```python
from build123d import *

# Parameters (mm, degrees)
SKETCH1_W                                            = 45
SKETCH1_H                                            = 50
SKETCH1_R                                            = 1.5
SKETCH1_R_2                                          = 2.5
BOSS_EXTRUDE1_DEPTH                                  = 20
SKETCH3_W                                            = 26
SKETCH3_H                                            = 28
CUT_EXTRUDE1_DEPTH                                   = 10
REFRENTADO_PARA_TORNILLO_CON_CABEZA_PLAN_D           = 3.2
REFRENTADO_PARA_TORNILLO_CON_CABEZA_PLAN_CBORE_D     = 6.5
REFRENTADO_PARA_TORNILLO_CON_CABEZA_PLAN_CBORE_DEPTH = 2
FILLET4_R                                            = 5
BOSS_EXTRUDE4_DEPTH                                  = 50
FILLET5_R                                            = 4.5
FILLET6_R                                            = 2.5


with BuildPart() as part:
    # Sketch1 → Boss-Extrude1 (new body)
    with BuildSketch(Plane(origin=(0, 0, 0), x_dir=(1, 0, 0), z_dir=(0, 1, 0))):
        Rectangle(SKETCH1_W, SKETCH1_H)
        with Locations(Location((-7.5, 8, 0), (0, 0, 270))):
            Circle(SKETCH1_R, mode=Mode.SUBTRACT)
        with Locations(Location((7.5, 8, 0), (0, 0, 270))):
            Circle(SKETCH1_R, mode=Mode.SUBTRACT)
        with Locations(Location((7.5, -8, 0), (0, 0, 270))):
            Circle(SKETCH1_R, mode=Mode.SUBTRACT)
        with Locations(Location((-7.5, -8, 0), (0, 0, 270))):
            Circle(SKETCH1_R, mode=Mode.SUBTRACT)
        with Locations(Location((15.3, 17, 0), (0, 0, 270))):
            Circle(SKETCH1_R_2, mode=Mode.SUBTRACT)
        with Locations(Location((-15.3, 17, 0), (0, 0, 270))):
            Circle(SKETCH1_R_2, mode=Mode.SUBTRACT)
        with Locations(Location((-15.3, -17, 0), (0, 0, 270))):
            Circle(SKETCH1_R_2, mode=Mode.SUBTRACT)
        with Locations(Location((15.3, -17, 0), (0, 0, 270))):
            Circle(SKETCH1_R_2, mode=Mode.SUBTRACT)
    extrude(amount=BOSS_EXTRUDE1_DEPTH)

    # Sketch3 → Cut-Extrude1 (cut)
    with BuildSketch(Plane(origin=(0, 20, 0), x_dir=(1, 0, 0), z_dir=(0, 1, 0))):
        Rectangle(SKETCH3_W, SKETCH3_H)
    extrude(amount=-CUT_EXTRUDE1_DEPTH, mode=Mode.SUBTRACT)

    # Refrentado para tornillo con cabeza plana de M32 (through all)
    with Locations(Plane(origin=(0, 10, 0), x_dir=(1, 0, 0), z_dir=(0, 1, 0))):
        with Locations((-7.5, 8), (-7.5, -8), (7.5, -8), (7.5, 8)):
            CounterBoreHole(REFRENTADO_PARA_TORNILLO_CON_CABEZA_PLAN_D / 2, REFRENTADO_PARA_TORNILLO_CON_CABEZA_PLAN_CBORE_D / 2, REFRENTADO_PARA_TORNILLO_CON_CABEZA_PLAN_CBORE_DEPTH)

    # Fillet4
    # the kernel refuses this fillet: 5 mm, written as the material it adds along each edge
    with BuildSketch(Plane(origin=(13, 10, 14), x_dir=(0, 1, 0), z_dir=(0, 0, -1))) as fillet4_piece_1_section:
        with BuildLine():
            CenterArc((FILLET4_R, -FILLET4_R), FILLET4_R, 90, 90)
            Line((0, -FILLET4_R), (0, 0))
            Line((0, 0), (FILLET4_R, 0))
        make_face()
    fillet4_piece_1 = extrude(amount=28, mode=Mode.PRIVATE)
    fillet4_piece_1 = fillet4_piece_1 - Plane(origin=(7.5, 11.149497573, 8), x_dir=(1, 0, 0), z_dir=(0, 1, 0)) * Cylinder(3.25, 76, mode=Mode.PRIVATE)
    fillet4_piece_1 = fillet4_piece_1 - Plane(origin=(7.5, 11.149497573, -8), x_dir=(1, 0, 0), z_dir=(0, 1, 0)) * Cylinder(3.25, 76, mode=Mode.PRIVATE)
    add(fillet4_piece_1)
    with BuildSketch(Plane(origin=(-13, 10, 14), x_dir=(0, 1, 0), z_dir=(1, 0, 0))) as fillet4_piece_2_section:
        with BuildLine():
            CenterArc((FILLET4_R, -FILLET4_R), FILLET4_R, 90, 90)
            Line((0, -FILLET4_R), (0, 0))
            Line((0, 0), (FILLET4_R, 0))
        make_face()
    fillet4_piece_2 = extrude(amount=26, mode=Mode.PRIVATE)
    fillet4_piece_2 = fillet4_piece_2 - Plane(origin=(-7.5, 11.135296279, 8), x_dir=(1, 0, 0), z_dir=(0, 1, 0)) * Cylinder(3.25, 72, mode=Mode.PRIVATE)
    fillet4_piece_2 = fillet4_piece_2 - Plane(origin=(7.5, 11.135296279, 8), x_dir=(1, 0, 0), z_dir=(0, 1, 0)) * Cylinder(3.25, 72, mode=Mode.PRIVATE)
    add(fillet4_piece_2)
    with BuildSketch(Plane(origin=(-13, 10, -14), x_dir=(0, 1, 0), z_dir=(0, 0, 1))) as fillet4_piece_3_section:
        with BuildLine():
            CenterArc((FILLET4_R, -FILLET4_R), FILLET4_R, 90, 90)
            Line((0, -FILLET4_R), (0, 0))
            Line((0, 0), (FILLET4_R, 0))
        make_face()
    fillet4_piece_3 = extrude(amount=28, mode=Mode.PRIVATE)
    fillet4_piece_3 = fillet4_piece_3 - Plane(origin=(-7.5, 11.149494803, 8), x_dir=(1, 0, 0), z_dir=(0, 1, 0)) * Cylinder(3.25, 76, mode=Mode.PRIVATE)
    fillet4_piece_3 = fillet4_piece_3 - Plane(origin=(-7.5, 11.149494803, -8), x_dir=(1, 0, 0), z_dir=(0, 1, 0)) * Cylinder(3.25, 76, mode=Mode.PRIVATE)
    add(fillet4_piece_3)
    with BuildSketch(Plane(origin=(13, 10, -14), x_dir=(0, 1, 0), z_dir=(-1, 0, 0))) as fillet4_piece_4_section:
        with BuildLine():
            CenterArc((FILLET4_R, -FILLET4_R), FILLET4_R, 90, 90)
            Line((0, -FILLET4_R), (0, 0))
            Line((0, 0), (FILLET4_R, 0))
        make_face()
    fillet4_piece_4 = extrude(amount=26, mode=Mode.PRIVATE)
    fillet4_piece_4 = fillet4_piece_4 - Plane(origin=(-7.5, 11.135296279, -8), x_dir=(1, 0, 0), z_dir=(0, 1, 0)) * Cylinder(3.25, 72, mode=Mode.PRIVATE)
    fillet4_piece_4 = fillet4_piece_4 - Plane(origin=(7.5, 11.135296279, -8), x_dir=(1, 0, 0), z_dir=(0, 1, 0)) * Cylinder(3.25, 72, mode=Mode.PRIVATE)
    add(fillet4_piece_4)

    # Sketch10 → Boss-Extrude4 (add, through all)
    with BuildSketch(Plane(origin=(0, 0, -25), x_dir=(-1, 0, 0), z_dir=(0, 0, -1))):
        Polygon((-15, 0), (-15, -24.067665252), (-19, -24.067665252), (-22.5, -14), (-22.5, 0), align=None)
    boss_extrude4 = extrude(amount=-BOSS_EXTRUDE4_DEPTH)

    # Mirror1: Boss-Extrude4 across plane
    add(boss_extrude4.mirror(Plane(origin=(0, 0, 0), x_dir=(0, 0, 1), z_dir=(1, 0, 0))))

    # Fillet5
    # the kernel refuses this fillet: 4.5 mm, written as the material it adds along each edge
    with BuildSketch(Plane(origin=(15, 0, -25.768065271), x_dir=(-1, 0, 0), z_dir=(0, 0, 1))) as fillet5_piece_1_section:
        with BuildLine():
            CenterArc((FILLET5_R, FILLET5_R), FILLET5_R, 180, 90)
            Line((0, FILLET5_R), (0, 0))
            Line((0, 0), (FILLET5_R, 0))
        make_face()
    fillet5_piece_1 = extrude(amount=51.536130542, mode=Mode.PRIVATE)
    fillet5_piece_1 = split(fillet5_piece_1, bisect_by=Plane(origin=(13.936107491, -0.973119841, 25), z_dir=(0, 0, -1)), keep=Keep.TOP, mode=Mode.PRIVATE)
    fillet5_piece_1 = fillet5_piece_1 - Plane(origin=(15.3, -0.973119841, 17), x_dir=(0, 0, 1), z_dir=(0, -1, 0)) * Cylinder(2.5, 122, mode=Mode.PRIVATE)
    fillet5_piece_1 = fillet5_piece_1 - Plane(origin=(15.3, -0.973119841, -17), x_dir=(0, 0, 1), z_dir=(0, -1, 0)) * Cylinder(2.5, 122, mode=Mode.PRIVATE)
    fillet5_piece_1 = split(fillet5_piece_1, bisect_by=Plane(origin=(13.936107491, -0.973119841, -25), z_dir=(0, 0, 1)), keep=Keep.TOP, mode=Mode.PRIVATE)
    add(fillet5_piece_1)
    with BuildSketch(Plane(origin=(-15, 0, -25.768065271), x_dir=(1, 0, 0), z_dir=(0, 0, 1))) as fillet5_piece_2_section:
        with BuildLine():
            CenterArc((FILLET5_R, -FILLET5_R), FILLET5_R, 90, 90)
            Line((0, -FILLET5_R), (0, 0))
            Line((0, 0), (FILLET5_R, 0))
        make_face()
    fillet5_piece_2 = extrude(amount=51.536130542, mode=Mode.PRIVATE)
    fillet5_piece_2 = fillet5_piece_2 - Plane(origin=(-15.3, -0.973119841, -17), x_dir=(0, 0, 1), z_dir=(0, -1, 0)) * Cylinder(2.5, 122, mode=Mode.PRIVATE)
    fillet5_piece_2 = fillet5_piece_2 - Plane(origin=(-15.3, -0.973119841, 17), x_dir=(0, 0, 1), z_dir=(0, -1, 0)) * Cylinder(2.5, 122, mode=Mode.PRIVATE)
    fillet5_piece_2 = split(fillet5_piece_2, bisect_by=Plane(origin=(-13.936107491, -0.973119841, 25), z_dir=(0, 0, -1)), keep=Keep.TOP, mode=Mode.PRIVATE)
    fillet5_piece_2 = split(fillet5_piece_2, bisect_by=Plane(origin=(-13.936107491, -0.973119841, -25), z_dir=(0, 0, 1)), keep=Keep.TOP, mode=Mode.PRIVATE)
    add(fillet5_piece_2)

    # Fillet6
    fillet6_edges = [part.edges().sort_by_distance(p)[0] for p in [
        (-22.5, 20, 0),
        (22.5, 20, 0),
    ]]
    fillet(fillet6_edges, radius=FILLET6_R)


solid = part.part
```
Verification items for the finished model (mm, model axes). A direction names the side the tool comes from. Coordinates: 2 decimals unless noted, no trailing zeros. Write each loop counter-clockwise with the first axis right and the second up, starting at its lowest first coordinate (ties: lowest second). Pieces come first, ordered by that corner, then holes. Notation, with made-up numbers: M 56.25,83 L 107.25,83 A17 ccw 107.25,98 Z; hole C 49,20 d4. An arc over 180 degrees is marked long. Answer as a JSON object with one key per item and string values. Group by question number.
(1) Release check for a two-part mould opening along Z. For faces 4 (the face through (-10.079, 9.118, 9.978)), 5 (the face through (-14, 20, 0)), 6 (the face through (0, 3, 25)) record: +Z half, -Z half, draft (parallel to the pull), parting line (faces both ways), or undercut.
(2) Cross-section at A-A, the plane y = 4.5. State how many separate pieces and enclosed holes the cut face has, and give its area (3 significant figures).
(3) Tool access check on faces 1 (the face through (16, 0, -17)), 2 (the face through (13.717, -1.353, -0.35)), 3 (the face through (20.726, -19.104, -0.35)). Record the directions out of +Z, -Z, +X, -X, +Y, -Y that give a thin tool (end or side, any length) a straight path to the whole face; none if there is none.
(4) Gauge pin test, flat ends, axial feed: pin 1 (3 mm diameter, centred on x = -7, z = -8.5, fed in from +Y); pin 2 (7.5 mm diameter, centred on x = -7.5, z = -8, fed in from +Y); pin 3 (1.4 mm diameter, centred on x = 16.5, z = -18, fed in from +Y). Record the tip position at first contact, or that the pin passes through.
(5) Cross-section at D-D, the plane y = -16.5. Record the cut outline in (x, z), and give its area (3 significant figures).
(6) Material ranges on line 1 (Z direction, x = -7.5, y = 6.5); line 2 (Z direction, x = -15.3, y = 2.25); line 3 (X direction, y = 12, z = 17), recorded low to high.
(7) Cross-section at B-B, the plane z = -17. Record the cut outline in (x, y).
(8) Cross-section at C-C, the plane x = -7. Record the cut outline in (y, z).
Reply:
{
 "1": {"face 4": "undercut", "face 5": "draft", "face 6": "+Z half"},
 "2": {"separate pieces": "1", "enclosed holes": "8", "area": "2,140 mm²"},
 "3": {"face 1": "+Y", "face 2": "+Z, -Z, -Y", "face 3": "+Z, -Z, +X, -Y"},
 "4": {"pin 1": "y = 8", "pin 2": "y = 11.2", "pin 3": "y = 0"},
 "5": {"outline": "M -21.63,-25 L -15,-25 L -15,25 L -21.63,25 Z; M 15,-25 L 21.63,-25 L 21.63,25 L 15,25 Z", "area": "663 mm²"},
 "6": {"line 1": "-25 to -9.6, -6.4 to 6.4, 9.6 to 25", "line 2": "-25 to -19.5, -14.5 to 14.5, 19.5 to 25", "line 3": "-22.5 to -17.8, -12.8 to 12.8, 17.8 to 22.5"},
 "7": {"outline": "M -22.5,-14 L -19,-24.07 L -15,-24.07 L -15,0 L -17.8,0 L -17.8,20 L -20,20 A2.5 ccw -22.5,17.5 Z; M -12.8,-0.63 A4.5 cw -10.5,0 L 10.5,0 A4.5 cw 12.8,-0.63 L 12.8,20 L -12.8,20 Z; M 15,-24.07 L 19,-24.07 L 22.5,-14 L 22.5,17.5 A2.5 ccw 20,20 L 17.8,20 L 17.8,0 L 15,0 Z"},
 "8": {"outline": "M 0,-25 L 20,-25 L 20,-14 L 15,-14 A5 cw 10.52,-11.21 L 8,-11.21 L 8,-9.52 L 0,-9.52 Z; M 0,-6.48 L 8,-6.48 L 8,-4.79 L 10,-4.79 L 10,4.79 L 8,4.79 L 8,6.48 L 0,6.48 Z; M 0,9.52 L 8,9.52 L 8,11.21 L 10.52,11.21 A5 cw 15,14 L 20,14 L 20,25 L 0,25 Z"}
}
